Geometry: final body of the model. Coordinates: model frame, mm. Face numbers are marked on the shaded views. A direction names the side the tool comes from. Give positions to 0.01 mm unless a question says otherwise; leave off trailing zeros. Loops run counter-clockwise (first coordinate to the right, second up) from the corner with the lowest first, then second, coordinate; pieces in that order, holes last.
from build123d import *

# Parameters (mm, degrees)
BOSS_EXTRUDE1_DEPTH = 15
CUT_EXTRUDE1_DEPTH  = 12
SKETCH4_W           = 21.61522369
SKETCH4_H           = 10.5
BOSS_EXTRUDE2_DEPTH = 12
CUT_EXTRUDE2_DEPTH  = 32.807611845
CUT_EXTRUDE4_START  = -17.615224
CUT_EXTRUDE4_DEPTH  = 17.615224


with BuildPart() as part:
    # Sketch2 → Boss-Extrude1 (new body)
    with BuildSketch(Plane(origin=(0, 0, 0), x_dir=(1, 0, 0), z_dir=(0, 1, 0))):
        Polygon((-21, 11.807611845), (-21, -11.807611845), (-11.807611845, -21), (11.807611845, -21), (21, -11.807611845), (21, 11.807611845), (11.807611845, 21), (-11.807611845, 21), align=None)
    extrude(amount=BOSS_EXTRUDE1_DEPTH)

    # Sketch3 → Cut-Extrude1 (cut)
    with BuildSketch(Plane(origin=(0, 15, 0), x_dir=(1, 0, 0), z_dir=(0, 1, 0))):
        Polygon((10.97918472, 19), (-10.97918472, 19), (-19, 10.97918472), (-19, -10.97918472), (-10.97918472, -19), (10.97918472, -19), (19, -10.97918472), (19, 10.97918472), align=None)
    extrude(amount=-CUT_EXTRUDE1_DEPTH, mode=Mode.SUBTRACT)

    # Sketch4 → Boss-Extrude2 (add)
    with BuildSketch(Plane.XY.offset(21)):
        with Locations((0, 6.75)):
            Rectangle(SKETCH4_W, SKETCH4_H)
    extrude(amount=BOSS_EXTRUDE2_DEPTH)

    # Sketch5 → Cut-Extrude2 (cut, through all)
    with BuildSketch(Plane(origin=(10.807611845, 0, 0), x_dir=(0, 0, -1), z_dir=(1, 0, 0))):
        Polygon((-25.331702881, 1.5), (-27.204226548, 2.702565985), (-27.204226548, 6.802747117), (-21, 10.304066646), (-21, 12), (-33, 12), (-33, 1.5), align=None)
    extrude(amount=-CUT_EXTRUDE2_DEPTH, mode=Mode.SUBTRACT)

    # Sketch6 → Cut-Extrude4 (cut)
    with BuildSketch(Plane(origin=(8.807611845, 0, 0), x_dir=(0, 0, -1), z_dir=(1, 0, 0)).offset(CUT_EXTRUDE4_START)):
        with BuildLine():
            Line((-27.204226548, 6.802747117), (-24.65218816, 8.242975286))
            ThreePointArc((-24.65218816, 8.242975286), (-22.383701286, 5.248553265), (-22.630570395, 1.5))
            Line((-22.630570395, 1.5), (-25.331702881, 1.5))
            ThreePointArc((-25.331702881, 1.5), (-24.594474047, 4.742322139), (-27.204226548, 6.802747117))
        make_face()
    extrude(amount=CUT_EXTRUDE4_DEPTH, mode=Mode.SUBTRACT)


solid = part.part
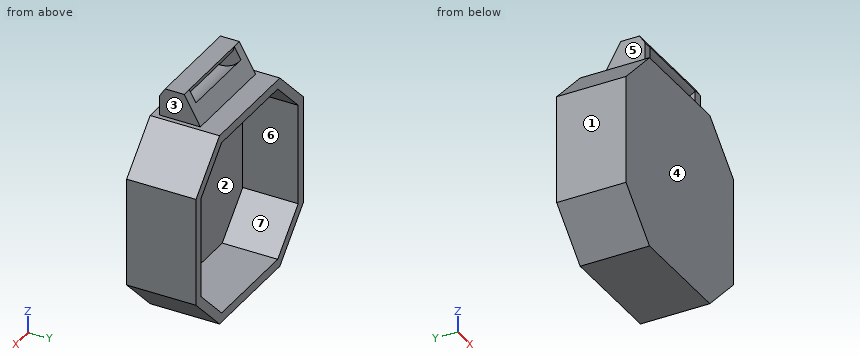
Item 1: Set-up query: the marked faces 1, 2 and 3. Return all of +Z, -Z, +X, -X, +Y, -Y with unobstructed straight access to the full face (end or side cutting, diameter ignored); none if empty.
Values follow:
face 1: +Z, -Z, -X, +Y, -Y
face 2: +Y
face 3: +Z, +X, +Y, -Y
Item 2: Ray query, probe 1 along X at (y, z) = (13.25, 5); probe 2 along Z at (x, y) = (10, 4.25). Return the intervals inside material, ascending.
Values follow:
probe 1: x = -21 to -19, 19 to 21
probe 2: z = -21 to -19, 19 to 27.2
Item 3: Section query C-C on x = 2. Return loops of the section in (y, z), plus the area to 3 significant figures.
Values follow:
outline: (0, -21) - (15, -21) - (15, -19) - (3, -19) - (3, 19) - (15, 19) - (15, 21) - (10.3, 21) - (8.24, 24.65) arc R5.37 cw to (1.5, 22.63) - (1.5, 21) - (0, 21) - close; (1.5, 25.33) arc R3.11 ccw to (6.8, 27.2) - (2.7, 27.2) - close
area: 200 mm2
Item 4: Section query A-A on y = 12.75. Return loops of the section in (x, z).
Values follow:
outline: (-21, -11.81) - (-11.81, -21) - (11.81, -21) - (21, -11.81) - (21, 11.81) - (11.81, 21) - (-11.81, 21) - (-21, 11.81) - close; hole (-19, -10.98) - (-10.98, -19) - (10.98, -19) - (19, -10.98) - (19, 10.98) - (10.98, 19) - (-10.98, 19) - (-19, 10.98) - close
Item 5: Section query B-B on z = -10. Return loops of the section in (x, y).
Values follow:
outline: (-21, 0) - (21, 0) - (21, 15) - (19, 15) - (19, 3) - (-19, 3) - (-19, 15) - (-21, 15) - close
Item 6: Pin query (flat end, axial travel): pin 1 (2.5 mm diameter, centred on y = 4, z = 24.5, fed in from -X); pin 2 (3 mm diameter, centred on y = 5, z = 25.5, fed in from +X); pin 3 (1.5 mm diameter, centred on x = 14, y = 12, fed in from +Z). Return the tip coordinate at first contact, or that it passes through.
Values follow:
pin 1: stops at x = -10.81
pin 2: stops at x = 10.81
pin 3: stops at z = 19.56
Item 7: Section query D-D on y = 6.25. Return loops of the section in (x, z).
Values follow:
outline: (-21, -11.81) - (-11.81, -21) - (11.81, -21) - (21, -11.81) - (21, 11.81) - (11.81, 21) - (10.81, 21) - (10.81, 27.2) - (-10.81, 27.2) - (-10.81, 21) - (-11.81, 21) - (-21, 11.81) - close; hole (-19, -10.98) - (-10.98, -19) - (10.98, -19) - (19, -10.98) - (19, 10.98) - (10.98, 19) - (-10.98, 19) - (-19, 10.98) - close; hole (-8.81, 22.8) - (8.81, 22.8) - (8.81, 25.74) - (-8.81, 25.74) - close
Item 8: Draft query along X for the marked faces 4, 5, 6 and 7. Return one class per face: +X half, -X half, draft (parallel to the pull), parting line (faces both ways), or undercut.
Values follow:
face 4: draft
face 5: -X half
face 6: undercut
face 7: undercut
